Build history of the part. All positions in model axes, mm. A direction names the side the tool comes from. Give positions to 0.01 mm unless a question says otherwise; leave off trailing zeros. Order: outer loops, then holes, each group sorted by start corner. A loop starts at its lowest first (then second) coordinate and runs counter-clockwise, first axis right, second up. Notation, with made-up numbers: (60, 7.25) -> (81, 7.25) arc R23 ccw to (81, 16.25) -> close; hole circle Ø8 at (-21.5, 38). An arc over 180 degrees is marked (long way). One line per item, written item: value. Start each with the question number.
(1) Two-plate mould, pull along Z, no slides. Class faces 5 (the flat face through (0, 50.546, 25)), 6 (the flat face through (0, 59, 29.272)), 7 (the cylindrical face through (0.043, 45.122, 158.945)), 8 (the flat face through (0, 75, 15.748)): +Z half, -Z half, draft (parallel to the pull), parting line (faces both ways), or undercut.
(2) Saw through at C-C on x = 1.25. Give the cut face in (y, z) (3 decimals), plus the area to 3 significant figures.
(3) Probe line 1 (Y direction, x = -0.25, z = 101); line 2 (Z direction, x = 0, y = 64.5); line 3 (Y direction, x = -1.5, z = 38). List the from-to ranges inside material, lowest first.
(4) Saw through at A-A on z = 13. Give the cut face in (x, y).
(5) Which spindle directions (+Z, -Z, +X, -X, +Y, -Y) get a long thin tool onto all of the face, cutting with end or side? Do faces 1 (the flat face through (0, 61, -45.72)), 2 (the flat face through (0, 77.978, 13)), 3 (the flat face through (0, 50.546, -42)), 4 (the flat face through (0, 55.626, 108)). Say none if no direction does.
(6) Saw through at B-B on y = 65. Give the cut face in (x, z).
(7) Pin check, flat tips, straight feed: pin 1 (3 mm diameter, centred on x = -1, y = 60, fed in from +Z); pin 2 (1.5 mm diameter, centred on x = 0, y = 47, fed in from -Z); pin 3 (1.8 mm diameter, centred on x = 0, z = 19.5, fed in from -Y); pin 4 (4 mm diameter, centred on y = 51.31, z = 147.86, fed in from +X). Stop position of each tip, or through.
(8) Saw through at D-D on z = 50. Give the cut face in (x, y), plus the area to 3 significant figures.
```python
from build123d import *

# Parameters (mm, degrees)
SKETCH1_R           = 3.175
SKETCH1_W           = 6.096
SKETCH1_H           = 6.35
BOSS_EXTRUDE1_DEPTH = 3.048


with BuildPart() as part:
    # Sketch1 → Boss-Extrude1 (new, symmetric)
    with BuildSketch(Plane(origin=(0, 0, 0), x_dir=(0, 0, -1), z_dir=(1, 0, 0))):
        with BuildLine():
            Line((-94.642365809, 55.626), (-122.457292876, 55.626))
            Line((-122.457292876, 55.626), (-122.457292876, 49.53))
            Line((-122.457292876, 49.53), (-142.309833129, 39.889958968))
            ThreePointArc((-142.309833129, 39.889958968), (-159.075906045, 45.361766519), (-154.207292876, 62.312827982))
            Line((-154.207292876, 62.312827982), (-113.876191878, 85.598))
            Line((-113.876191878, 85.598), (20.203427503, 85.598))
            Line((20.203427503, 85.598), (45.72, 70.866))
            Line((45.72, 70.866), (45.72, 50.546))
            Line((45.72, 50.546), (38.1, 50.546))
            Line((38.1, 50.546), (38.1, 55.626))
            Line((38.1, 55.626), (-9.652, 55.626))
            Line((-9.652, 55.626), (-9.652, 61.976))
            Line((-9.652, 61.976), (-15.748, 61.976))
            Line((-15.748, 61.976), (-15.748, 55.626))
            Line((-15.748, 55.626), (-21.651856626, 55.626))
            Line((-21.651856626, 55.626), (-21.651856626, 50.546))
            Line((-21.651856626, 50.546), (-29.271856626, 50.546))
            Line((-29.271856626, 50.546), (-29.271856626, 68.326))
            Line((-29.271856626, 68.326), (-87.022365809, 68.326))
            Line((-87.022365809, 68.326), (-87.022365809, 49.022))
            Line((-87.022365809, 49.022), (-94.642365809, 49.022))
            Line((-94.642365809, 49.022), (-94.642365809, 55.626))
        make_face()
        with Locations((-147.857292876, 51.314305354)):
            Circle(SKETCH1_R, mode=Mode.SUBTRACT)
        with Locations((-12.7, 74.803)):
            Rectangle(SKETCH1_W, SKETCH1_H, mode=Mode.SUBTRACT)
    extrude(amount=BOSS_EXTRUDE1_DEPTH, both=True)


solid = part.part
```
Results below:
1. face 5: draft
1. face 6: undercut
1. face 7: parting line
1. face 8: undercut
2. outline: (39.89, 142.31) -> (49.53, 122.457) -> (55.626, 122.457) -> (55.626, 94.642) -> (49.022, 94.642) -> (49.022, 87.022) -> (68.326, 87.022) -> (68.326, 29.272) -> (50.546, 29.272) -> (50.546, 21.652) -> (55.626, 21.652) -> (55.626, 15.748) -> (61.976, 15.748) -> (61.976, 9.652) -> (55.626, 9.652) -> (55.626, -38.1) -> (50.546, -38.1) -> (50.546, -45.72) -> (70.866, -45.72) -> (85.598, -20.203) -> (85.598, 113.876) -> (62.313, 154.207) arc R12.7 ccw to start; hole circle Ø6.35 at (51.314, 147.857); hole (71.628, 9.652) -> (77.978, 9.652) -> (77.978, 15.748) -> (71.628, 15.748) -> close
2. area: 5,130 mm²
3. line 1: y = 55.63 to 85.6
3. line 2: z = -45.72 to 29.27, 87.02 to 150.42
3. line 3: y = 68.33 to 85.6
4. outline: (-3.05, 61.98) -> (3.05, 61.98) -> (3.05, 71.63) -> (-3.05, 71.63) -> close; (-3.05, 77.98) -> (3.05, 77.98) -> (3.05, 85.6) -> (-3.05, 85.6) -> close
5. face 1: -Z, +X, -X, +Y, -Y
5. face 2: +X, -X
5. face 3: -Z, +X, -X, -Y
5. face 4: +X, -X, -Y
6. outline: (-3.05, -45.72) -> (3.05, -45.72) -> (3.05, 29.27) -> (-3.05, 29.27) -> close; (-3.05, 87.02) -> (3.05, 87.02) -> (3.05, 149.55) -> (-3.05, 149.55) -> close
7. pin 1: stops at z = 158.33
7. pin 2: stops at z = 126.12
7. pin 3: stops at y = 55.63
7. pin 4: passes through
8. outline: (-3.05, 68.33) -> (3.05, 68.33) -> (3.05, 85.6) -> (-3.05, 85.6) -> close
8. area: 105 mm²
